Autodesk Inventor part; units mm, degrees
ref_plane "Work Plane1" through (0, 0, 139.7) normal (0, 0, 1) x (1, 0, 0)
ref_plane "Work Plane2" through (0, 215.9, -34.98) normal (0, 0, 1) x (1, 0, 0)
ref_plane "YZ Plane" through (0, 0, 0) normal (1, 0, 0) x (0, 1, 0)
sketch "Sketch2" plane through (0, 0, 0) normal (0, 0, 1) x (1, 0, 0)
  line L0 (0, 0) -> (0, 304.8)
  line L1 (30.98, 0) -> (30.98, 215.9)
  line L2 (30.98, 215.9) -> (107.18, 215.9)
  line L3 (107.18, 215.9) -> (62.73, 0)
  line L4 (62.73, 0) -> (30.98, 0)
  line L5 (105.9531, 214.9) -> (31.98, 214.9)
  line L6 (31.98, 214.9) -> (31.98, 1)
  line L7 (31.98, 1) -> (61.9149, 1)
  line L8 (61.9149, 1) -> (105.9531, 214.9)
  dimension "d2" = 304.8
  dimension "d3" = 30.98
  dimension "d4" = 76.2
  dimension "d5" = 31.75
  dimension "d7" = 215.9
  dimension "d8" = 0
  dimension "d9" = 1
revolve "Revolution1" add sketch "Sketch2" angle 360 about axis through (0, 0, 0) along (0, 1, 0)
ref_plane "Work Plane1" through (0, 0, 139.7) normal (0, 0, 1) x (1, 0, 0)
sketch "Sketch3" plane through (0, 0, 139.7) normal (0, 0, 1) x (1, 0, 0)
  circle A0 centre (0, 177.8) radius 3
  line L0 (107.18, 215.9) -> (-107.18, 215.9)
  line L1 (0, 0) -> (0, 215.9)
  dimension "d12" = 6
  dimension "d13" = 38.1
extrude "Extrusion1" cut sketch "Sketch3" against normal blind 52.3875
pattern_circular "Circular Pattern1" count 3 over 360 about axis through (0, 107.95, 0) along (0, 1, 0) of "Extrusion1"
sketch "Sketch4" plane through (0, 215.9, 0) normal (0, 1, 0) x (1, 0, 0)
  circle A0 centre (0, 0) radius 30.98
  circle A1 centre (0, 0) radius 30.98
  circle A2 centre (0, 0) radius 34.98
  dimension "d19" = 4
extrude "Extrusion2" add sketch "Sketch4" along normal blind 8.89
ref_plane "Work Plane2" through (0, 215.9, -34.98) normal (0, 0, 1) x (1, 0, 0)
sketch "Sketch5" plane through (0, 215.9, -34.98) normal (0, 0, 1) x (1, 0, 0)
  line L0 (-30.98, 8.89) -> (30.98, 8.89)
  line L1 (107.18, 0) -> (-107.18, 0)
  line L2 (3.27, 8.89) -> (1.27, 8.89)
  line L3 (1.27, 8.89) -> (1.27, 0)
  line L4 (1.27, 0) -> (3.27, 0)
  line L5 (3.27, 0) -> (3.27, 8.89)
  line L6 (-1.27, 8.89) -> (-3.27, 8.89)
  line L7 (-3.27, 8.89) -> (-3.27, 0)
  line L8 (-3.27, 0) -> (-1.27, 0)
  line L9 (-1.27, 0) -> (-1.27, 8.89)
  line L10 (0, 8.89) -> (0, 0)
  point P0 (0, -215.9)
  point P1 (3.27, 0)
  point P2 (1.27, 8.89)
  point P3 (-1.27, 0)
  point P4 (-1.27, 8.89)
  point P5 (-3.27, 8.89)
  point P6 (-3.27, 0)
  dimension "d22" = 2
  dimension "d24" = 2.54
extrude "Extrusion3" add sketch "Sketch5" along normal blind 2.54 and the other way blind 5.08 contours L0 L9 L1 L7 | L0 L5 L1 L3
sketch "Sketch7" plane through (0, 215.9, -34.98) normal (0, 0, 1) x (1, 0, 0)
  line L0 (1.27, 0) -> (1.27, 8.89)
  line L1 (-30.98, 8.89) -> (30.98, 8.89)
  line L2 (1.27, 0) -> (-1.27, 0)
  line L3 (-1.27, 0) -> (-1.27, 8.89)
  line L4 (-1.27, 8.89) -> (1.27, 8.89)
  line L5 (1.27, 8.89) -> (1.27, 0)
  line L6 (-1.27, 8.89) -> (-1.27, 0)
  point P0 (0, -215.9)
  dimension "d29" = 0
extrude "Extrusion4" cut sketch "Sketch7" along normal up to surface
sketch "Sketch8" plane through (3.27, 215.9, -34.8268) normal (1, 0, 0) x (0, 0, -1)
  line L0 (0, 8.89) -> (5.2332, 8.89)
  line L1 (2.6932, 8.89) -> (2.6932, 0)
  line L2 (72.3532, 0) -> (-142.0068, 0)
  line L3 (5.2332, 8.89) -> (5.2332, 0)
  circle A0 centre (2.6932, 6.985) radius 1.27
  circle A1 centre (2.6932, 3.175) radius 1.27
  point P0 (-34.8268, -215.9)
  dimension "d32" = 0
  dimension "d33" = 2.54
  dimension "d37" = 2.54
  dimension "d38" = 2.54
  dimension "d39" = 1.905
  dimension "d40" = 3.81
sketch "Sketch9" plane through (0, 215.9, -40.06) normal (0, 0, -1) x (-1, 0, 0)
  line L0 (1.27, 0) -> (1.27, 8.89)
  line L1 (34.98, 0) -> (34.98, 8.89)
  line L2 (1.27, 0) -> (34.98, 0)
  line L3 (34.98, 0) -> (34.98, 1)
  line L4 (34.98, 1) -> (1.27, 1)
  line L5 (1.27, 1) -> (1.27, 0)
  point P0 (0, -215.9)
  point P1 (1.27, 1)
  dimension "d34" = 1
extrude "Extrusion5" cut sketch "Sketch9" against normal blind 101.6
extrude "Extrusion6" cut sketch "Sketch8" against normal up to surface (6.54 mm away) contours A0 L1 | L1 A0 | A1 L1 | L1 A1
properties part number "Water Sensor Bouy 4_3DPrint"
Input: part model. Units: mm. Frame: model coordinates. A direction names the side the tool comes from. Round coordinates to 2 decimals unless told otherwise and drop trailing zeros. Write each loop counter-clockwise with the first axis right and the second up, starting at its lowest first coordinate (ties: lowest second). Pieces come first, ordered by that corner, then holes.
1) Cut plane A-A (z = 0). Return the cut outline in (x, y).
2) Draft query along Y for faces 5 (the flat face through (-1.27, 221, -36)), 6 (the cylindrical face through (-3, 177.9, 98.8)), 7 (the flat face through (-29, 0, 13)), 8 (the flat face through (-8, 224.79, -31)). Return one class per face: pulls with the +Y half, pulls with the -Y half, needs draft (parallel to the pull), parting line crosses it, or undercut.
3) Cut plane C-C (x = 24). Count the separate pieces of the cut face and the enclosed holes in it, then the cut area to 3 significant figures.
4) Ray query, L1, parallel to Y at x = -1.95, z = -37.52 (3 decimals); L2, parallel to Y at x = -1, z = -37; L3, parallel to Y at x = 4.5, z = -32. Return the intervals inside material, ascending.
5) Reachability of faces 1 (the cylindrical face through (23.065, 220.283, 26.298)), 2 (the flat face through (-31, 216.9, -6)), 3 (the flat face through (1.27, 220, -36)), 4 (the conical face through (75.7, 85.7, -23.8)) from +Z, -Z, +X, -X, +Y, -Y: full face, straight path, thin tool, end or side. Return the list, or none.
6) Cut plane B-B (y = 24). Return the cut outline in (x, z).
7) Contact query for flat-ended pins moving along their axis: P1, Ø1.1, axis at y = 216, z = 32.5, coming from the -X side; P2, Ø1, axis at y = 123, z = 31.5, coming from the -X side; P3, Ø4, axis at x = 74.5, y = 133, coming from the +Z side; P4, Ø1.5, axis at y = 222.885, z = -37.52, coming from the -X side. Output: stop coordinate, or through.
Geometry says:
1. outline: (-107.18, 215.9) - (-62.73, 0) - (-30.98, 0) - (-30.98, 215.9) - close; (-34.98, 216.9) - (-30.98, 216.9) - (-30.98, 224.79) - (-34.98, 224.79) - close; (30.98, 0) - (62.73, 0) - (107.18, 215.9) - (34.98, 215.9) - (34.98, 224.79) - (30.98, 224.79) - close; hole (-105.95, 214.9) - (-61.91, 1) - (-31.98, 1) - (-31.98, 214.9) - close; hole (31.98, 1) - (61.91, 1) - (105.95, 214.9) - (31.98, 214.9) - close
2. face 5: needs draft
2. face 6: undercut
2. face 7: pulls with the -Y half
2. face 8: pulls with the +Y half
3. separate pieces: 2
3. enclosed holes: 2
3. area: 1,470 mm2
4. L1: y = 0 to 1, 214.9 to 215.9, 216.9 to 217.805, 220.345 to 221.615, 224.155 to 224.79
4. L2: y = 0 to 1, 214.9 to 215.9
4. L3: y = 0 to 1, 214.9 to 224.79
5. face 1: +Y
5. face 2: +Z, -Z, -X
5. face 3: -Z, +Y
5. face 4: none
6. outline: circle Ø135.34 at (0, 0); circle Ø63.96 at (0, 0); hole circle Ø133.3 at (0, 0); hole circle Ø61.96 at (0, 0)
7. P1: stops at x = -102.3
7. P2: stops at x = -82.45
7. P3: stops at z = 53.6
7. P4: passes through
